from build123d import *

# Parameters (mm, degrees)
F0_R     = 50
F1_DEPTH = 3
F2_DEPTH = 35
F3_DEPTH = 32
F4_DEPTH = 84.6
F5_DEPTH = 25


with BuildPart() as f1:
    # F0 (on Top) → F1 (new body)
    with BuildSketch(Plane.XY):
        with BuildLine():
            ThreePointArc((65, 1.5318503138), (31.467850574, 58.406927283), (-34.5315193925, 56.600663343))
            ThreePointArc((-34.5315193925, 56.600663343), (-56.5003016989, 33.6677478107), (-64.98194699, 3.0637006275))
            Line((-64.98194699, 3.0637006275), (-64.98194699, 0))
            ThreePointArc((-64.98194699, 0), (0.7659783442, -63.463636277), (65, 1.5318503138))
        make_face()
        Circle(F0_R, mode=Mode.SUBTRACT)
        Circle(F0_R)
        with BuildLine():
            Line((-70, -70), (70, -70))
            Line((70, -70), (70, 70))
            Line((70, 70), (-34.5315193925, 70))
            Line((-34.5315193925, 70), (-34.5315193925, 56.600663343))
            ThreePointArc((-34.5315193925, 56.600663343), (31.467850574, 58.406927283), (65, 1.5318503138))
            ThreePointArc((65, 1.5318503138), (0.7659783442, -63.463636277), (-64.98194699, 0))
            ThreePointArc((-64.98194699, 0), (-65, 1.5318503138), (-64.98194699, 3.0637006275))
            Line((-64.98194699, 3.0637006275), (-64.98194699, 70))
            Line((-64.98194699, 70), (-70, 70))
            Line((-70, 70), (-70, -70))
        make_face()
        with BuildLine():
            Line((-34.5315193925, 56.600663343), (-34.5315193925, 70))
            Line((-34.5315193925, 70), (-64.98194699, 70))
            Line((-64.98194699, 70), (-64.98194699, 3.0637006275))
            ThreePointArc((-64.98194699, 3.0637006275), (-56.5003016989, 33.6677478107), (-34.5315193925, 56.600663343))
        make_face()
        with BuildLine():
            Line((-64.98194699, 0), (-64.98194699, 3.0637006275))
            ThreePointArc((-64.98194699, 3.0637006275), (-65, 1.5318503138), (-64.98194699, 0))
        make_face()
    extrude(amount=-F1_DEPTH)

    # F2 (add): a face of the model
    f2_faces = [f1.faces().sort_by_distance(p)[0] for p in [
        (0, 0, 0),
    ]]
    extrude(f2_faces, amount=F2_DEPTH)

    # F0 (on Top) → F3 (cut)
    with BuildSketch(Plane.XY):
        with BuildLine():
            ThreePointArc((65, 1.5318503138), (31.467850574, 58.406927283), (-34.5315193925, 56.600663343))
            ThreePointArc((-34.5315193925, 56.600663343), (-56.5003016989, 33.6677478107), (-64.98194699, 3.0637006275))
            Line((-64.98194699, 3.0637006275), (-64.98194699, 0))
            ThreePointArc((-64.98194699, 0), (0.7659783442, -63.463636277), (65, 1.5318503138))
        make_face()
        Circle(F0_R, mode=Mode.SUBTRACT)
        Circle(F0_R)
        with BuildLine():
            Line((-34.5315193925, 56.600663343), (-34.5315193925, 70))
            Line((-34.5315193925, 70), (-64.98194699, 70))
            Line((-64.98194699, 70), (-64.98194699, 3.0637006275))
            ThreePointArc((-64.98194699, 3.0637006275), (-56.5003016989, 33.6677478107), (-34.5315193925, 56.600663343))
        make_face()
    extrude(amount=F3_DEPTH, mode=Mode.SUBTRACT)

    # F0 (on Top) → F4 (cut)
    with BuildSketch(Plane.XY):
        Circle(F0_R)
    extrude(amount=F4_DEPTH, mode=Mode.SUBTRACT)

    # F0 (on Top) → F5 (cut)
    with BuildSketch(Plane.XY):
        Circle(F0_R)
    extrude(amount=-F5_DEPTH, mode=Mode.SUBTRACT)


solid = f1.part
Design review of the part built by this model. Coordinates are the model's own, in mm. A direction names the side the tool comes from. Coordinates: 2 decimals unless noted, no trailing zeros. Loops run counter-clockwise (first coordinate to the right, second up) from the corner with the lowest first, then second, coordinate; pieces in that order, holes last. Notation, with made-up numbers: M -26.5,1.25 L 10.5,1.25 A19 ccw 10.5,34.25 Z; hole C 7,73 d4. An arc over 180 degrees is marked long. Use one line per item in the form item = value.
(1) For faces 5 (the face through (-34.532, 63, 16)), 6 (the face through (-15, 49, 0)), 7 (the face through (-48, 17, 35)), list the 3-axis set-ups (+Z, -Z, +X, -X, +Y, -Y) from which the entire face can be reached by the end or side of a thin tool; tool diameter is ignored.
Return value:
face_5 = +Y
face_6 = none
face_7 = +Z, +X, -X, +Y, -Y
(2) Consider section D-D (x = 61). Write out the cut boundary in (y, z), and give its area (3 significant figures).
Return value:
outline = M -70,-3 L 70,-3 L 70,35 L -70,35 Z; hole M -20.92,0 L 23.98,0 L 23.98,32 L -20.92,32 Z
area = 3,880 mm2
(3) Consider section A-A (x = 0). Write out the cut boundary in (y, z), and give its area (3 significant figures).
Return value:
outline = M -70,-3 L -50,-3 L -50,0 L -63.47,0 L -63.47,32 L -50,32 L -50,35 L -70,35 Z; M 50,-3 L 70,-3 L 70,35 L 50,35 L 50,32 L 66.53,32 L 66.53,0 L 50,0 Z
area = 560 mm2
(4) Draft analysis for pull direction X (two halves, no side actions). For faces 1 (the face through (70, -1, 16)), 2 (the face through (-1, -70, 16)), 3 (the face through (-64.982, 35, 16)), 4 (the face through (-70, 1, 16)), state which applies: pulls with the +X half, pulls with the -X half, needs draft (parallel to the pull), parting line crosses it, or undercut.
Return value:
face_1 = pulls with the +X half
face_2 = needs draft
face_3 = undercut
face_4 = pulls with the -X half
(5) Consider section B-B (y = -26.5). Write out the cut boundary in (x, z).
Return value:
outline = M -70,-3 L -42.4,-3 L -42.4,0 L -58.64,0 L -58.64,32 L -42.4,32 L -42.4,35 L -70,35 Z; M 42.4,-3 L 70,-3 L 70,35 L 42.4,35 L 42.4,32 L 58.64,32 L 58.64,0 L 42.4,0 Z
(6) For line 1 along Y through (x, z) = (0, -1); line 2 along Y through (x, z) = (0, 13); line 3 along Z through (x, y) = (44.5, 36), list the stretches that pass through material, from the lowest coordinate up. Write a range as from..to.
Return value:
line_1 = -70..-50, 50..70
line_2 = -70..-63.47, 66.53..70
line_3 = -3..0, 32..35
(7) Consider section C-C (z = 20). Write out the cut boundary in (x, y).
Return value:
outline = M -70,-70 L 70,-70 L 70,70 L -34.53,70 L -34.53,56.6 A65 cw long -64.98,0 L -64.98,70 L -70,70 Z
